```python
from build123d import *

# Parameters (mm, degrees)
F0_W     = 140
F0_H     = 50
F1_DEPTH = 10
F2_W     = 10
F2_H     = 50
F3_DEPTH = 70
F4_R     = 5
F5_DEPTH = 140.001
F6_W     = 140.089303
F6_H     = 159.690752
F7_DEPTH = 50.001


with BuildPart() as f1:
    # F0 (on Front) → F1 (new body)
    with BuildSketch(Plane.XZ):
        Rectangle(F0_W, F0_H)
    extrude(amount=F1_DEPTH)

    # F2 (on face) → F3 (join)
    with BuildSketch(Plane(origin=(0, 0, 0), x_dir=(-1, 0, 0), z_dir=(0, 1, 0))):
        with Locations((-65, 0)):
            Rectangle(F2_W, F2_H)
        with Locations((65, 0)):
            Rectangle(F2_W, F2_H)
    extrude(amount=F3_DEPTH)

    # F4 (on face) → F5 (cut, through all)
    with BuildSketch(Plane(origin=(-70, 0, 0), x_dir=(0, -1, 0), z_dir=(-1, 0, 0))):
        with Locations((-60, 0)):
            Circle(F4_R)
    extrude(amount=-F5_DEPTH, mode=Mode.SUBTRACT)

    # F6 (on face) → F7 (cut, through all)
    with BuildSketch(Plane(origin=(0, 0, -25), x_dir=(1, 0, 0), z_dir=(0, 0, -1))):
        with Locations((70.044652, -4.198499)):
            Rectangle(F6_W, F6_H)
    extrude(amount=-F7_DEPTH, mode=Mode.SUBTRACT)


solid = f1.part
```
Build history of the part. All positions in model axes, mm. A direction names the side the tool comes from. Round coordinates to 2 decimals unless told otherwise and drop trailing zeros. Write each loop counter-clockwise with the first axis right and the second up, starting at its lowest first coordinate (ties: lowest second). Pieces come first, ordered by that corner, then holes. Notation, with made-up numbers: (-4.75, 49) - (25.25, 49) arc R20 ccw to (25.25, 73) - close; hole circle Ø1 at (71.5, -28.75). An arc over 180 degrees is marked (long way). Answer as CSV lines item,"result".
Q1. Drop flat-ended pins along their axis: pin 1 (25 mm diameter, centred on y = 28.5, z = 10.5, fed in from +X); pin 2 (1 mm diameter, centred on x = -48.5, z = 14, fed in from +Y); pin 3 (8 mm diameter, centred on y = 60, z = 0, fed in from +X). Give the stop position or say it passes through.
Report:
pin 1,"stops at x = -60"
pin 2,"stops at y = 0"
pin 3,"passes through"
Q2. Cut at A-A (z = 0). Write the cut outline in (x, y).
Report:
outline,"(-70, -10) - (0, -10) - (0, 0) - (-60, 0) - (-60, 55) - (-70, 55) - close; (-70, 65) - (-60, 65) - (-60, 70) - (-70, 70) - close"
Q3. Cut at D-D (z = -9.5). Write the cut outline in (x, y), and give its area (3 significant figures).
Report:
outline,"(-70, -10) - (0, -10) - (0, 0) - (-60, 0) - (-60, 70) - (-70, 70) - close"
area,"1,400 mm^2"
Q4. Cut at B-B (y = 60). Write the cut outline in (x, z).
Report:
outline,"(-70, -25) - (-60, -25) - (-60, -5) - (-70, -5) - close; (-70, 5) - (-60, 5) - (-60, 25) - (-70, 25) - close"
Q5. Tool access for faces 1 (the flat face through (-30, 0, 0)), 2 (the flat face through (-70, 31, 0)): list every direction of +Z, -Z, +X, -X, +Y, -Y with a clear straight run to the whole face (end or side of a thin tool).
Report:
face 1,"+Z, -Z, +X, +Y"
face 2,"+Z, -Z, -X, +Y, -Y"
Q6. Drill centre lines: probe 1 along Z at (x, y) = (-64.5, 60); probe 2 along X at (y, z) = (8.5, 13.5); probe 3 along Y at (x, z) = (-9, -4). Where is each one in solid material? Low to high. Write a range as [from, to].
Report:
probe 1,"z = [-25, -5], [5, 25]"
probe 2,"x = [-70, -60]"
probe 3,"y = [-10, 0]"
Q7. Cut at C-C (x = -61). Write the cut outline in (y, z), and give its area (3 significant figures).
Report:
outline,"(-10, -25) - (70, -25) - (70, 25) - (-10, 25) - close; hole circle Ø10 at (60, 0)"
area,"3,920 mm^2"
Q8. Pull direction Z, two halves, no side cores. Call faces 3 (the flat face through (-61, 15, -25)), 4 (the cylindrical face through (-65, 65, 0)), 5 (the flat face through (-35, -10, 0)): +Z half, -Z half, draft (parallel to the pull), parting line (faces both ways), or undercut.
Report:
face 3,"-Z half"
face 4,"undercut"
face 5,"draft"
